Verification items for the finished model (mm, model axes). A direction names the side the tool comes from. Coordinates: 2 decimals unless noted, no trailing zeros. Order: outer loops, then holes, each group sorted by start corner. A loop starts at its lowest first (then second) coordinate and runs counter-clockwise, first axis right, second up.
Q1. Cross-section at B-B, the plane x = 0.4. Record the boundary of the cut face in (y, z), and give its area (3 significant figures).
Q2. Cross-section at A-A, the plane z = 3.75. Record the boundary of the cut face in (x, y).
Q3. Thickness scan on line 1 (X direction, y = 11, z = 4.5); line 2 (Y direction, x = 1.1, z = 3.5); line 3 (Y direction, x = 1.45, z = 0.5). Record the ranges inside material, lowest first.
Q4. Set-up check for faces 1 (the flat face through (0.8, 6, 0)), 2 (the flat face through (-0.8, 7, 0)): record each of +Z, -Z, +X, -X, +Y, -Y from which the full face is reachable in a straight line by a thin tool's end or side.
Q5. Cross-section at C-C, the plane y = 8. Record the boundary of the cut face in (x, z), and give its area (3 significant figures).
Autodesk Inventor part; units mm, degrees
ref_plane "YZ Plane" through (0, 0, 0) normal (1, 0, 0) x (0, 1, 0)
ref_plane "XZ Plane" through (0, 0, 0) normal (0, 1, 0) x (-1, 0, 0)
ref_plane "XY Plane" through (0, 0, 0) normal (0, 0, 1) x (1, 0, 0)
sketch "Sketch1" plane through (0, 0, 0) normal (0, 1, 0) x (-1, 0, 0)
  line L0 (-0.8, -5) -> (0.8, -5)
  line L1 (0.8, -5) -> (0.8, 5)
  line L2 (0.8, 5) -> (-0.8, 5)
  line L3 (-0.8, 5) -> (-0.8, -5)
  line L4 (-0.8, -5) -> (0.8, 5) construction
  line L5 (0.8, -5) -> (-0.8, 5) construction
  point P0 (0, 0)
  dimension "length" = 10
  dimension "width" = 1.6
extrude "Extrusion1" add sketch "Sketch1" along normal blind 12.65
sketch "Sketch3" plane through (-0.8, 0, 5) normal (0, 0, 1) x (1, 0, 0)
  line L0 (1.6, 12.65) -> (2.4, 12.65)
  line L1 (1.6, 0) -> (1.6, 12.65)
  line L2 (2.4, 12.65) -> (2.4, 13.05)
  line L3 (0, 13.85) -> (0.4, 13.85)
  line L4 (2.4, 13.05) -> (0.4, 13.85)
  line L5 (0, 0) -> (0, 12.65)
  line L6 (0, 0) -> (0, 12.65)
  line L7 (0, 13.85) -> (0, 12.65)
  line L8 (0, 12.65) -> (1.6, 12.65)
  line L9 (1.6, 0) -> (1.6, 12.65)
  point P0 (0.8, 0)
  dimension "fixer" = 0.8
  dimension "d8" = 0.4
  dimension "d11" = 0.4
  dimension "d12" = 1.2
extrude "Extrusion2" add sketch "Sketch3" against normal blind 10
equation "\"d6\" = length"
equation "\"TOL\" = 0.15"
properties part number "straight"
Check values:
1. outline: (0, -5) - (13.53, -5) - (13.53, 5) - (0, 5) - close
1. area: 135 mm2
2. outline: (-0.8, 0) - (0.8, 0) - (0.8, 12.65) - (1.6, 12.65) - (1.6, 13.05) - (-0.4, 13.85) - (-0.8, 13.85) - close
3. line 1: x = -0.8 to 0.8
3. line 2: y = 12.65 to 13.25
3. line 3: y = 12.65 to 13.11
4. face 1: +Z, -Z, +X, -Y
4. face 2: +Z, -Z, -X, +Y, -Y
5. outline: (-0.8, -5) - (0.8, -5) - (0.8, 5) - (-0.8, 5) - close
5. area: 16.0 mm2
